```python
from build123d import *

# Parameters (mm, degrees)
CROQUIS1_W               = 9
CROQUIS1_H               = 31.5
CROQUIS1_R               = 2.25
SALIENTE_EXTRUIR1_DEPTH  = 1.5
CROQUIS11_W              = 24
CROQUIS11_H              = 24
CROQUIS11_W_2            = 20
CROQUIS11_H_2            = 20
SALIENTE_EXTRUIR8_DEPTH  = 15
SALIENTE_EXTRUIR11_DEPTH = 3


with BuildPart() as part:
    # Croquis1 → Saliente-Extruir1 (new, symmetric)
    with BuildSketch(Plane.XY):
        with Locations((0, 10.15)):
            Rectangle(CROQUIS1_W, CROQUIS1_H)
        Circle(CROQUIS1_R, mode=Mode.SUBTRACT)
    extrude(amount=SALIENTE_EXTRUIR1_DEPTH, both=True)

    # Croquis11 → Saliente-Extruir8 (add, symmetric)
    with BuildSketch(Plane.XY):
        with Locations((0, 35.9)):
            Rectangle(CROQUIS11_W, CROQUIS11_H)
        with Locations((0, 35.9)):
            Rectangle(CROQUIS11_W_2, CROQUIS11_H_2, mode=Mode.SUBTRACT)
    extrude(amount=SALIENTE_EXTRUIR8_DEPTH, both=True)

    # Croquis13 → Saliente-Extruir11 (add, symmetric)
    with BuildSketch(Plane(origin=(0, 0, 0), x_dir=(0, 0, -1), z_dir=(1, 0, 0))):
        Polygon((1.5, 10.95), (1.5, 23.9), (7.5, 23.9), align=None)
        Polygon((-7.5, 23.9), (-1.5, 10.95), (-1.5, 23.9), align=None)
    extrude(amount=SALIENTE_EXTRUIR11_DEPTH, both=True)


solid = part.part
```
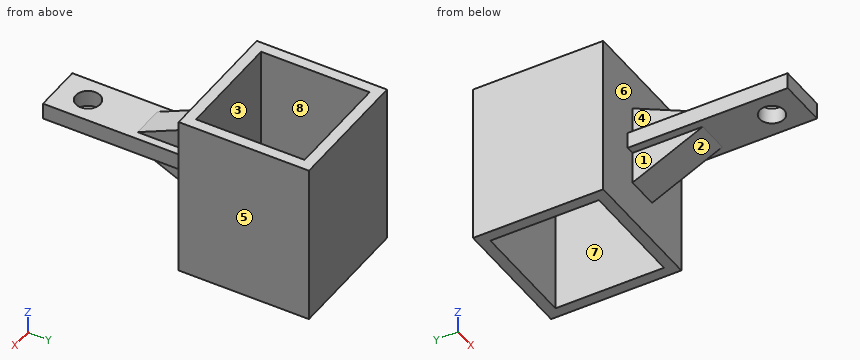
Input: part model. Units: mm. Frame: model coordinates. Face numbers are marked on the shaded views. A direction names the side the tool comes from. Give positions to 0.01 mm unless a question says otherwise; leave off trailing zeros. Order: outer loops, then holes, each group sorted by start corner. A loop starts at its lowest first (then second) coordinate and runs counter-clockwise, first axis right, second up. Notation, with made-up numbers: M 86,35.5 L 118,35.5 A10 cw 118,50.5 Z; hole C 88.5,-17 d7. An arc over 180 degrees is marked long. Return JSON: item names as keys, results as strings.
1) Section query A-A on y = 0. Output: boundary loops of the cut face in (x, z).
Taken from the geometry:
{"outline": "M -4.5,-1.5 L -2.25,-1.5 L -2.25,1.5 L -4.5,1.5 Z; M 2.25,-1.5 L 4.5,-1.5 L 4.5,1.5 L 2.25,1.5 Z"}
2) Contact query for flat-ended pins moving along their axis: pin 1 (2.5 mm diameter, centred on x = -0.5, y = 6, fed in from +Z); pin 2 (2 mm diameter, centred on x = 4.5, z = -11, fed in from -Y); pin 3 (2.5 mm diameter, centred on x = 0, y = 8, fed in from -Z); pin 4 (4 mm diameter, centred on x = 0, y = 0, fed in from -Z). Output: stop coordinate, or through.
Taken from the geometry:
{"pin 1": "stops at z = 1.5", "pin 2": "stops at y = 23.9", "pin 3": "stops at z = -1.5", "pin 4": "passes through"}
3) Mould query, pull axis X, two halves, no side actions, for the marked faces 5, 6, 7 and 8. Classes: released by +X, released by -X, zero draft, split by the parting line, or undercut.
Taken from the geometry:
{"face 5": "released by +X", "face 6": "zero draft", "face 7": "undercut", "face 8": "undercut"}
4) Line query: L1, parallel to Y at x = 0, z = 0.55; L2, parallel to Y at x = -0.5, z = -10.75; L3, parallel to X at y = 36, z = 6.5. Output: solid intervals per line, ascending. Write a range as [from, to].
Taken from the geometry:
{"L1": "y = [-5.6, -2.25], [2.25, 25.9], [45.9, 47.9]", "L2": "y = [23.9, 25.9], [45.9, 47.9]", "L3": "x = [-12, -10], [10, 12]"}
5) Access query for the marked faces 1, 2, 3 and 4. Directions: +Z, -Z, +X, -X, +Y, -Y. A direction counts if a zero-diameter tool reaches every point of the face in a straight line with its end or side. Return the directions, or none.
Taken from the geometry:
{"face 1": "-Z, -X, -Y", "face 2": "-Z, +X, -X, -Y", "face 3": "+Z, -Z", "face 4": "+Z, -X, -Y"}
6) Section query B-B on z = -10.25. Output: boundary loops of the cut face in (x, y).
Taken from the geometry:
{"outline": "M -12,23.9 L 12,23.9 L 12,47.9 L -12,47.9 Z; hole M -10,25.9 L 10,25.9 L 10,45.9 L -10,45.9 Z"}
7) Section query C-C on x = 0. Output: boundary loops of the cut face in (y, z).
Taken from the geometry:
{"outline": "M -5.6,-1.5 L -2.25,-1.5 L -2.25,1.5 L -5.6,1.5 Z; M 2.25,-1.5 L 10.95,-1.5 L 23.9,-7.5 L 23.9,-15 L 25.9,-15 L 25.9,15 L 23.9,15 L 23.9,7.5 L 10.95,1.5 L 2.25,1.5 Z; M 45.9,-15 L 47.9,-15 L 47.9,15 L 45.9,15 Z"}
8) Section query D-D on x = 8.5. Output: boundary loops of the cut face in (y, z).
Taken from the geometry:
{"outline": "M 23.9,-15 L 25.9,-15 L 25.9,15 L 23.9,15 Z; M 45.9,-15 L 47.9,-15 L 47.9,15 L 45.9,15 Z"}
